Could you check a few things on this model? Use its own coordinates, in mm. A direction names the side the tool comes from. Coordinates: 2 decimals unless noted, no trailing zeros. Loops run counter-clockwise (first coordinate to the right, second up) from the corner with the lowest first, then second, coordinate; pieces in that order, holes last.
1) Thinking about a two-plate mould opening in Z: for faces 4 (the face through (32.667, 36.712, 32.684)), 5 (the face through (9, 23, -36)), 6 (the face through (31.018, 34.958, 30.468)), which applies, released by +Z, released by -Z, zero draft, split by the parting line, or undercut?
2) If I drill on line 1 along X through (y, z) = (35, 29.5); line 2 along X through (y, z) = (38, 16); line 3 along X through (y, z) = (23.5, -32), over which ranges is the centre line in solid material (lowest first)?
3) Will these pins go through, and if not, where does the flat tip stop? P1, Ø6, axis at x = -2.5, z = 30, coming from the +Y side; P2, Ø3.5, axis at x = -4, z = 24, coming from the +Y side; P3, Ø12.5, axis at x = -29, y = 29.5, coming from the -Z side; P4, Ø3, axis at x = 29.5, z = -1.5, coming from the +Y side.
4) For faces 1 (the face through (-3, 38, 28)), 2 (the face through (-21.2, 6.7, 7.4)), 3 (the face through (-8, 16, 11)), which set-ups out of +Z, -Z, +X, -X, +Y, -Y let a thin tool reach every point of the face, with its end or its side?
5) Imagine slicing it at A-A on y = 10. Please give me the cut outline in (x, z).
6) Imagine slicing it at B-B on y = 20. Give the number of separate pieces and of enclosed holes in the cut face, plus the area to 3 significant figures.
```python
from build123d import *

# Parameters (mm, degrees)
SKETCH1_W           = 72
SKETCH1_H           = 72
SKETCH1_R           = 12
SKETCH1_R_2         = 1.8
BOSS_EXTRUDE1_DEPTH = 40
SKETCH6_W           = 44
SKETCH6_H           = 44
CUT_EXTRUDE1_DEPTH  = 32
CHAMFER1_SIZE       = 18
SKETCH7_W           = 18
SKETCH7_H           = 18
CUT_EXTRUDE2_DEPTH  = 65.745656225
CHAMFER2_SIZE       = 8
CHAMFER3_SIZE       = 4
SKETCH8_R           = 3
CUT_EXTRUDE3_DEPTH  = 2
CHAMFER5_SIZE       = 6
CHAMFER6_SIZE       = 6
CHAMFER7_SIZE       = 12
SKETCH9_R           = 2.1
CUT_EXTRUDE4_DEPTH  = 6
SKETCH10_R          = 2.1
CUT_EXTRUDE5_DEPTH  = 6
SKETCH11_R          = 8.15
CUT_EXTRUDE6_DEPTH  = 5
FILLET1_R           = 2
SKETCH13_R          = 6.75
CUT_EXTRUDE7_DEPTH  = 1
SKETCH15_R          = 2.1
CUT_EXTRUDE8_DEPTH  = 6
CHAMFER8_SIZE       = 1
SKETCH16_W          = 11.455844123
SKETCH16_H          = 76.568397014
CUT_EXTRUDE9_DEPTH  = 8
SKETCH17_W          = 86.001258557
SKETCH17_H          = 11.455844123
CUT_EXTRUDE10_DEPTH = 8
CHAMFER9_SIZE       = 3


with BuildPart() as part:
    # Sketch1 → Boss-Extrude1 (new body)
    with BuildSketch(Plane(origin=(0, 0, 0), x_dir=(1, 0, 0), z_dir=(0, 1, 0))):
        Rectangle(SKETCH1_W, SKETCH1_H)
        with Locations(Location((14, -14, 0), (0, 0, 270))):
            Circle(SKETCH1_R, mode=Mode.SUBTRACT)
        with Locations(Location((29.5, 1.5, 0), (0, 0, 270))):
            Circle(SKETCH1_R_2, mode=Mode.SUBTRACT)
        with Locations(Location((29.5, -29.5, 0), (0, 0, 270))):
            Circle(SKETCH1_R_2, mode=Mode.SUBTRACT)
        with Locations(Location((-1.5, -29.5, 0), (0, 0, 270))):
            Circle(SKETCH1_R_2, mode=Mode.SUBTRACT)
        with Locations(Location((-1.5, 1.5, 0), (0, 0, 270))):
            Circle(SKETCH1_R_2, mode=Mode.SUBTRACT)
    extrude(amount=BOSS_EXTRUDE1_DEPTH)

    # Sketch6 → Cut-Extrude1 (cut)
    with BuildSketch(Plane(origin=(0, 0, 0), x_dir=(-1, 0, 0), z_dir=(0, -1, 0))):
        with Locations((-14, -14)):
            Rectangle(SKETCH6_W, SKETCH6_H)
    extrude(amount=-CUT_EXTRUDE1_DEPTH, mode=Mode.SUBTRACT)

    # Chamfer1
    chamfer1_edges = [part.edges().sort_by_distance(p)[0] for p in [
        (-36, 0, 0),
        (0, 0, -36),
        (-36, 20, -36),
    ]]
    chamfer(chamfer1_edges, length=CHAMFER1_SIZE)

    # Sketch7 → Cut-Extrude2 (cut, through all)
    with BuildSketch(Plane(origin=(0, 40, 0), x_dir=(1, 0, 0), z_dir=(0, 1, 0))):
        with Locations((-27, 27)):
            Rectangle(SKETCH7_W, SKETCH7_H)
    extrude(amount=-CUT_EXTRUDE2_DEPTH, mode=Mode.SUBTRACT)

    # Chamfer2
    # the kernel refuses this chamfer: 8 mm, written as the material it adds along each edge
    with BuildSketch(Plane(origin=(-18, 40, -18), x_dir=(0.027495876610586487, 0, -0.9996219169112968), z_dir=(0, -1, 0))) as chamfer2_piece_1_section:
        Polygon((CHAMFER2_SIZE * 0.999621916911, -CHAMFER2_SIZE * 0.0274958766106), (-CHAMFER2_SIZE * 0.0274958766106, -CHAMFER2_SIZE * 0.999621916911), (0, 0), align=None)
    chamfer2_piece_1 = extrude(amount=60.573463904, mode=Mode.PRIVATE)
    chamfer2_piece_1 = split(chamfer2_piece_1, bisect_by=Plane(origin=(-20.597865647, 12.296786874, -30.296786874), z_dir=(0, 0.7071067811865476, 0.7071067811865476)), keep=Keep.TOP, mode=Mode.PRIVATE)
    chamfer2_piece_1 = split(chamfer2_piece_1, bisect_by=Plane(origin=(-30.296786874, 12.296786874, -20.597865647), z_dir=(0.7071067811865476, 0.7071067811865476, 0)), keep=Keep.TOP, mode=Mode.PRIVATE)
    add(chamfer2_piece_1)

    # Chamfer3
    chamfer3_edges = [part.edges().sort_by_distance(p)[0] for p in [
        (36, 36, 36),
    ]]
    chamfer(chamfer3_edges, length=CHAMFER3_SIZE)

    # Sketch8 → Cut-Extrude3 (cut)
    with BuildSketch(Plane(origin=(0, 40, 0), x_dir=(1, 0, 0), z_dir=(0, 1, 0))):
        with Locations(Location((-1.5, 1.5, 0), (0, 0, 270))):
            Circle(SKETCH8_R)
        with Locations(Location((29.5, 1.5, 0), (0, 0, 270))):
            Circle(SKETCH8_R)
        with Locations(Location((29.5, -29.5, 0), (0, 0, 270))):
            Circle(SKETCH8_R)
        with Locations(Location((-1.5, -29.5, 0), (0, 0, 270))):
            Circle(SKETCH8_R)
    extrude(amount=-CUT_EXTRUDE3_DEPTH, mode=Mode.SUBTRACT)

    # Chamfer5
    chamfer5_edges = [part.edges().sort_by_distance(p)[0] for p in [
        (36, 16, -8),
        (-8, 16, 36),
    ]]
    chamfer(chamfer5_edges, length=CHAMFER5_SIZE)

    # Chamfer6
    # the kernel refuses this chamfer: 6 mm, written as the material it takes off along each edge
    with BuildSketch(Plane(origin=(36, 40, -51.430097928), x_dir=(0.027495876610586768, -0.9996219169112968, 0), z_dir=(0, 0, 1)), Plane(origin=(47.430097928, 40, 36), x_dir=(0, -0.9996219169112965, 0.02749587661058676), z_dir=(-1, 0, 0))) as chamfer6_piece_1:
        Polygon((CHAMFER6_SIZE * 0.999621916911, -CHAMFER6_SIZE * 0.0274958766106), (-CHAMFER6_SIZE * 0.0274958766106, -CHAMFER6_SIZE * 0.999621916911), (0, 0), align=None)
    extrude(amount=98.860195856, mode=Mode.SUBTRACT)

    # Chamfer7
    chamfer7_edges = [part.edges().sort_by_distance(p)[0] for p in [
        (6, 40, -36),
        (-36, 40, 6),
    ]]
    chamfer(chamfer7_edges, length=CHAMFER7_SIZE)

    # Sketch9 → Cut-Extrude4 (cut)
    with BuildSketch(Plane(origin=(0, -9, -9), x_dir=(-1, 0, 0), z_dir=(0, -0.7071067811865488, -0.7071067811865464))):
        with Locations(Location((11.977430497, 15.455844123, 0), (0, 0, 90))):
            Circle(SKETCH9_R)
        with Locations(Location((-20.022569503, 15.455844123, 0), (0, 0, 90))):
            Circle(SKETCH9_R)
        with Locations(Location((-20.022569503, 35.455844123, 0), (0, 0, 90))):
            Circle(SKETCH9_R)
        with Locations(Location((11.977430497, 35.455844123, 0), (0, 0, 90))):
            Circle(SKETCH9_R)
    extrude(amount=-CUT_EXTRUDE4_DEPTH, mode=Mode.SUBTRACT)

    # Sketch10 → Cut-Extrude5 (cut)
    with BuildSketch(Plane(origin=(-9, -9, 0), x_dir=(-0.7071067811865488, 0.7071067811865464, 0), z_dir=(-0.7071067811865464, -0.7071067811865488, 0))):
        with Locations(Location((35.455844123, 12, 0), (0, 0, 180))):
            Circle(SKETCH10_R)
        with Locations(Location((35.455844123, -20, 0), (0, 0, 180))):
            Circle(SKETCH10_R)
        with Locations(Location((15.455844123, -20, 0), (0, 0, 180))):
            Circle(SKETCH10_R)
        with Locations(Location((15.455844123, 12, 0), (0, 0, 180))):
            Circle(SKETCH10_R)
    extrude(amount=-CUT_EXTRUDE5_DEPTH, mode=Mode.SUBTRACT)

    # Sketch11 → Cut-Extrude6 (cut)
    with BuildSketch(Plane(origin=(0, 40, 0), x_dir=(1, 0, 0), z_dir=(0, 1, 0))):
        with Locations(Location((-4, 4, 0), (0, 0, 270))):
            Circle(SKETCH11_R)
    extrude(amount=-CUT_EXTRUDE6_DEPTH, mode=Mode.SUBTRACT)

    # Fillet1
    fillet1_edges = [part.edges().sort_by_distance(p)[0] for p in [
        (14, 40, 2),
        (14, 32, 2),
    ]]
    fillet(fillet1_edges, radius=FILLET1_R)

    # Sketch13 → Cut-Extrude7 (cut)
    with BuildSketch(Plane(origin=(0, 35, 0), x_dir=(1, 0, 0), z_dir=(0, 1, 0))):
        with Locations(Location((-4, 4, 0), (0, 0, 270))):
            Circle(SKETCH13_R)
    extrude(amount=-CUT_EXTRUDE7_DEPTH, mode=Mode.SUBTRACT)

    # Sketch15 → Cut-Extrude8 (cut)
    with BuildSketch(Plane(origin=(0, 40, 0), x_dir=(1, 0, 0), z_dir=(0, 1, 0))):
        with Locations(Location((16, 4, 0), (0, 0, 270))):
            Circle(SKETCH15_R)
        with Locations(Location((24, 4, 0), (0, 0, 270))):
            Circle(SKETCH15_R)
        with Locations(Location((-4, -16, 0), (0, 0, 270))):
            Circle(SKETCH15_R)
        with Locations(Location((-4, -24, 0), (0, 0, 270))):
            Circle(SKETCH15_R)
    extrude(amount=-CUT_EXTRUDE8_DEPTH, mode=Mode.SUBTRACT)

    # Chamfer8
    chamfer8_edges = [part.edges().sort_by_distance(p)[0] for p in [
        (-25, 39, -19),
        (-19, 39, -25),
        (33, 37, -27),
        (32.810660172, 37.189339828, 32.810660172),
        (-27, 37, 33),
    ]]
    chamfer(chamfer8_edges, length=CHAMFER8_SIZE)

    # Sketch16 → Cut-Extrude9 (cut)
    with BuildSketch(Plane(origin=(-9, -9, 0), x_dir=(-0.7071067811865488, 0.7071067811865464, 0), z_dir=(-0.7071067811865464, -0.7071067811865488, 0))):
        with Locations((25.455844123, 2.284198507)):
            Rectangle(SKETCH16_W, SKETCH16_H)
    extrude(amount=-CUT_EXTRUDE9_DEPTH, mode=Mode.SUBTRACT)

    # Sketch17 → Cut-Extrude10 (cut)
    with BuildSketch(Plane(origin=(0, -9, -9), x_dir=(-1, 0, 0), z_dir=(0, -0.7071067811865488, -0.7071067811865464))):
        with Locations((7.000629278, 25.455844123)):
            Rectangle(SKETCH17_W, SKETCH17_H)
    extrude(amount=-CUT_EXTRUDE10_DEPTH, mode=Mode.SUBTRACT)

    # Chamfer9
    chamfer9_edges = [part.edges().sort_by_distance(p)[0] for p in [
        (8.696699141, 18.707106781, -25.393398282),
        (-25.393398282, 18.707106781, 8.696699141),
        (9.353553391, 10.606601718, -17.292893219),
        (-17.292893219, 10.606601718, 9.353553391),
    ]]
    chamfer(chamfer9_edges, length=CHAMFER9_SIZE)


solid = part.part
```
Filled in:
1. face 4: released by +Z
1. face 5: released by -Z
1. face 6: undercut
2. line 1: x = -29 to -3.3, 0.3 to 27.7, 31.3 to 35
2. line 2: x = -26 to -6.1, -1.9 to 2.17, 25.83 to 32
2. line 3: x = -18 to 36
3. P1: stops at y = 40
3. P2: stops at y = 34
3. P3: stops at z = -21.25
3. P4: passes through
4. face 1: +Y
4. face 2: +Z, -Z, -X
4. face 3: +Z, +X, -Y
5. outline: (-19.41, -19.41) - (36, -19.41) - (36, -14) - (30, -8) - (-8, -8) - (-8, 30) - (-14, 36) - (-19.41, 36) - close
6. separate pieces: 1
6. enclosed holes: 4
6. area: 2,870 mm2
